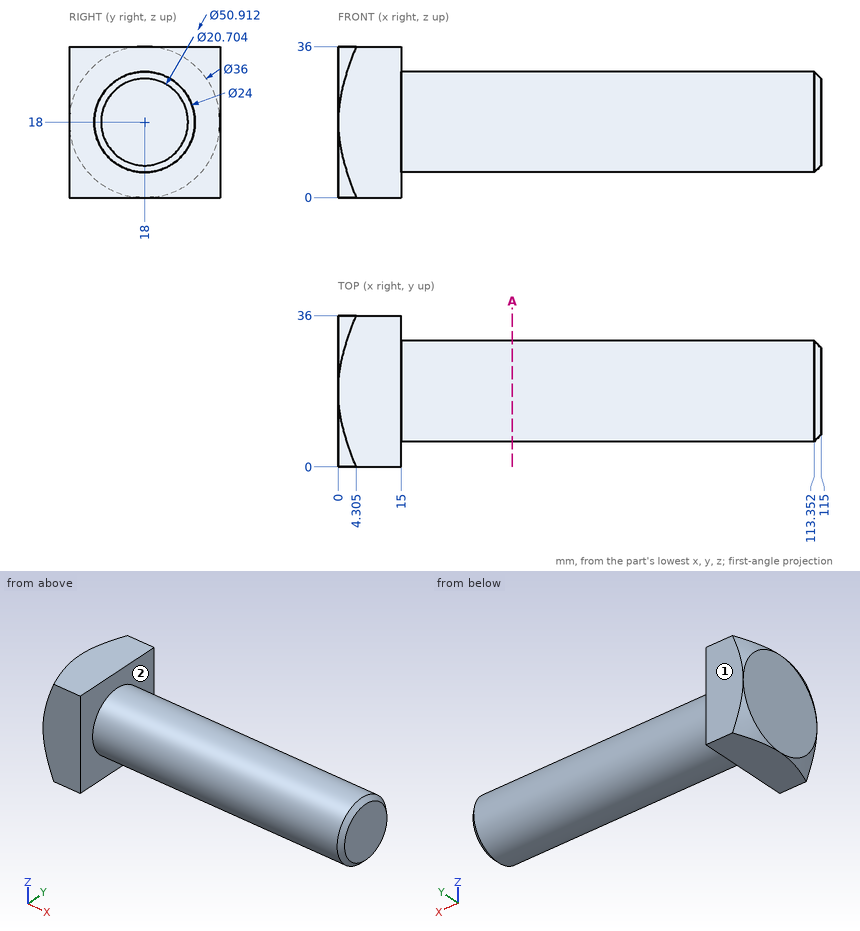
Geometry check sheet. Reference: drawing and pictorial views, mm from the part's lowest x, y, z. A direction names the side the tool comes from. Round coordinates to 2 decimals unless told otherwise and drop trailing zeros. Loops run counter-clockwise (first coordinate to the right, second up) from the corner with the lowest first, then second, coordinate; pieces in that order, holes last. Notation, with made-up numbers: (19, -14.75) - (25, -14.75) arc R29 ccw to (25, 6.25) - close; hole circle Ø1 at (-36, -16.75). An arc over 180 degrees is marked (long way). One line per question, with ' | ' between items. Start each with the question number.
1. Depth check by flat-ended pin: pin 1 (3 mm diameter, centred on x = 84.5, y = 16, fed in from -Z); pin 2 (3 mm diameter, centred on x = 24, z = 20, fed in from +Y); pin 3 (2 mm diameter, centred on x = 43, y = 29.5, fed in from -Z); pin 4 (6 mm diameter, centred on y = 25.5, z = 30.5, fed in from -X). Enter the tip coordinate at first touch or a pass-through.
2. Cross-section at A-A on x = 41.5. Record the cut outline in (y, z).
3. Tool access check on the marked faces 1 and 2. Record the directions out of +Z, -Z, +X, -X, +Y, -Y that give a thin tool (end or side, any length) a straight path to the whole face; none if there is none.
4. Scan lines: line 1 (Y direction, x = 19, z = 18.5); line 2 (X direction, y = 20.5, z = 2.5); line 3 (Z direction, x = 61, y = 17). Record each from-to range of solid material in increasing order. Write a range as [from, to].
Taken from the geometry:
1) pin 1: z = 6.01 | pin 2: y = 29.99 | pin 3: z = 12.19 | pin 4: x = 0
2) outline: circle Ø24 at (18, 18)
3) face 1: +Z, -Z, +X, -X, +Y | face 2: +X
4) line 1: [6.01, 29.99] | line 2: [0, 15] | line 3: [6.04, 29.96]
